Geometry: see drawing. Coordinates: mm, zero at the bounding-box minimum. Coordinates: 2 decimals unless noted, no trailing zeros. Write each loop counter-clockwise with the first axis right and the second up, starting at its lowest first coordinate (ties: lowest second). Pieces come first, ordered by that corner, then holes. Notation, with made-up numbers: (-16.5, -22) - (20.5, -22) arc R20 cw to (20.5, -11) - close; hole circle Ø7 at (18, 56.25). An arc over 180 degrees is marked (long way). Use a Markdown table: item, result. Add a question column.
Q1. Pin query (flat end, axial travel): P1, Ø3, axis at x = 147, y = 13, coming from the -Z side. Return the tip coordinate at first contact, or that it passes through.
Q2. Material intervals for probe 1 along X at (y, z) = (19.5, 4.5); probe 2 along Y at (x, z) = (71.5, 5.5); probe 3 along Z at (x, y) = (86.5, 10.25), sorted ascending. Write a range as from..to.
Q3. Section query A-A (x = 237). Return the cut outline in (y, z), then the cut area to 3 significant figures.
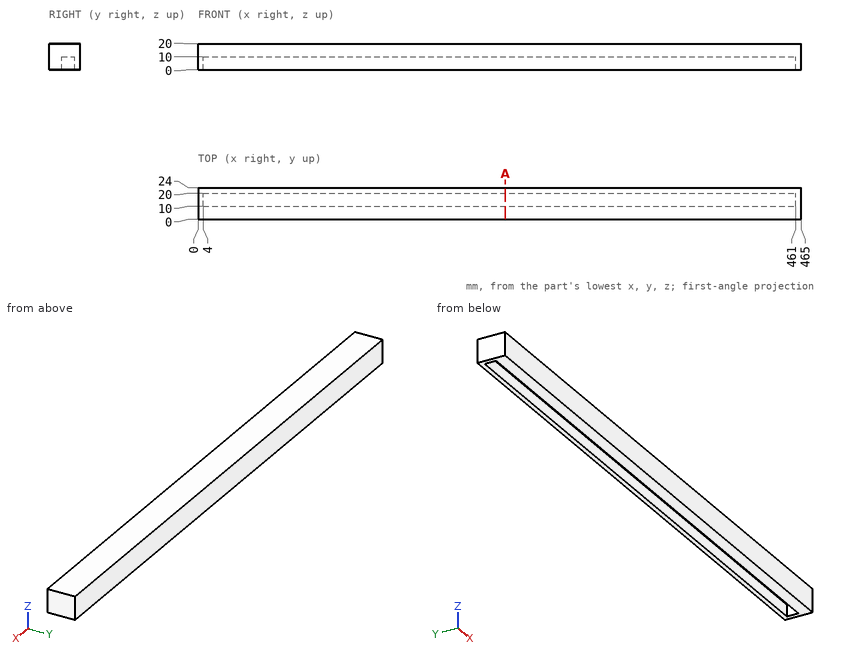
Values follow:
| question | item | result |
|---|---|---|
| 1 | P1 | z = 10 |
| 2 | probe 1 | 0..4, 461..465 |
| 2 | probe 2 | 0..10, 20..24 |
| 2 | probe 3 | 10..20 |
| 3 | outline | (0, 0) - (10, 0) - (10, 10) - (20, 10) - (20, 0) - (24, 0) - (24, 20) - (0, 20) - close |
| 3 | area | 380 mm2 |
